from build123d import *

# Parameters (mm, degrees)
SKETCH3_R         = 12.7
GEARBODY_DEPTH    = 6.35
TOOTHCUT_DEPTH    = 7.35
CIRPATTERN1_COUNT = 18
BORE_DEPTH        = 12.7


with BuildPart() as part:
    # Sketch3 → gearBody (new body)
    with BuildSketch(Plane.XY):
        Circle(SKETCH3_R)
    extrude(amount=GEARBODY_DEPTH)

    # Sketch2 → toothCut (cut, through all)
    with BuildSketch(Plane.XY):
        with BuildLine():
            ThreePointArc((9.781229257, -1.205205904), (9.806057787, -0.982953571), (9.825836884, -0.760195085))
            ThreePointArc((9.825836884, -0.760195085), (9.980803767, -0.435792976), (10.31355819, -0.299682883))
            ThreePointArc((10.31355819, -0.299682883), (12.38209996, 0.246018063), (13.970369973, 1.679214819))
            ThreePointArc((13.970369973, 1.679214819), (14.000763839, -1.403428484), (13.359117821, -4.418706897))
            ThreePointArc((13.359117821, -4.418706897), (12.0869153, -2.698778026), (10.167842346, -1.753360882))
            ThreePointArc((10.167842346, -1.753360882), (9.868724138, -1.553912241), (9.781229257, -1.205205904))
        make_face()
    toothcut = extrude(amount=TOOTHCUT_DEPTH, mode=Mode.SUBTRACT)

    # CirPattern1: toothCut ×18 about axis
    cirpattern1_axis = Axis((0, 0, 0), (0, 0, 1))
    for i in range(1, CIRPATTERN1_COUNT):
        add(toothcut.rotate(cirpattern1_axis, i * 360 / CIRPATTERN1_COUNT), mode=Mode.SUBTRACT)

    # boreDia → bore (cut, symmetric)
    with BuildSketch(Plane.XY):
        with BuildLine():
            Line((-1, 3.842012337), (-1, 4.992632337))
            Line((-1, 4.992632337), (1, 4.992632337))
            Line((1, 4.992632337), (1, 3.842012337))
            ThreePointArc((1, 3.842012337), (0, -3.97002), (-1, 3.842012337))
        make_face()
    extrude(amount=BORE_DEPTH, both=True, mode=Mode.SUBTRACT)


solid = part.part
Verification items for the finished model (mm, model axes). A direction names the side the tool comes from. Round coordinates to 2 decimals unless told otherwise and drop trailing zeros. Loops run counter-clockwise (first coordinate to the right, second up) from the corner with the lowest first, then second, coordinate; pieces in that order, holes last. Notation, with made-up numbers: (24, -28) - (41, -28) arc R24 ccw to (41, 6) - close; hole circle Ø3 at (73, 84.25). An arc over 180 degrees is marked (long way). Use a Markdown table: item, result. Add a question column.
1. Section check A-A, the plane y = 0. Record the boundary of the cut face in (x, z), plus the area to 3 significant figures.
2. Release check for a two-part mould opening along X. For faces 6 (the face through (-5.677, 10.045, 3.131)), 7 (the face through (-5.519, -11.438, 3.131)), 8 (the face through (7.146, -10.499, 3.131)) record: released by +X, released by -X, zero draft, split by the parting line, or undercut.
3. Thickness scan on probe 1 along X at (y, z) = (-11, 1.25); probe 2 along X at (y, z) = (-2.25, 1); probe 3 along Y at (x, z) = (-2.25, 4). Record the ranges inside material, lowest first. Write a range as [from, to].
4. Access from +Z, -Z, +X, -X, +Y, -Y to the whole of each face (thin tool, end or side, straight path). Record for faces 1 (the face through (-7.59, -8.74, 3.13)), 2 (the face through (-3.772, 10.939, 3.131)), 3 (the face through (-11.36, 2.203, 3.131)), 4 (the face through (4.14, 10.8, 3.13)), 5 (the face through (11.36, -2.203, 3.131)).
5. Gauge pin test, flat ends, axial feed: pin 1 (3 mm diameter, centred on x = 10, z = 1.5, fed in from -Y); pin 2 (1 mm diameter, centred on x = -5.5, z = 5, fed in from +Y); pin 3 (5 mm diameter, centred on x = 0, y = 0, fed in from -Z); pin 4 (3 mm diameter, centred on x = 7, z = 5.5, fed in from +Y). Record the tip position at first contact, or that the pin passes through.
Checks:
| question | item | result |
|---|---|---|
| 1 | outline | (-11.85, 0) - (-3.97, 0) - (-3.97, 6.35) - (-11.85, 6.35) - close; (3.97, 0) - (11.85, 0) - (11.85, 6.35) - (3.97, 6.35) - close |
| 1 | area | 100 mm^2 |
| 2 | face 6 | undercut |
| 2 | face 7 | released by -X |
| 2 | face 8 | released by +X |
| 3 | probe 1 | x = [-5.98, -4.31], [-2.14, -0.04], [1.73, 3.77] |
| 3 | probe 2 | x = [-9.59, -3.27], [3.27, 11.44] |
| 3 | probe 3 | y = [-9.65, -3.27], [3.27, 11.96] |
| 4 | face 1 | +Z, -Z, -Y |
| 4 | face 2 | +Z, -Z |
| 4 | face 3 | +Z, -Z, -X |
| 4 | face 4 | +Z, -Z, +Y |
| 4 | face 5 | +Z, -Z, +X |
| 5 | pin 1 | stops at y = -7.83 |
| 5 | pin 2 | stops at y = 10.32 |
| 5 | pin 3 | passes through |
| 5 | pin 4 | stops at y = 11.45 |
